```python
from build123d import *

# Parameters (mm, degrees)
F1_DEPTH = 31.75
F2_R     = 4.75
F3_DEPTH = 38.1
F5_D     = 4.572
F5_DEPTH = 7.621
F7_DEPTH = 12.7
F9_D     = 2
F11_D    = 5


# Not quite as in the source:
# - a feature names something its author has since deleted; it is built from what else it names


with BuildPart() as f1:
    # F0 (on Top) → F1 (new body)
    with BuildSketch(Plane.XY):
        with BuildLine():
            Line((-7.62, 10.9198254229), (-7.62, 0))
            ThreePointArc((-7.62, 0), (0, -7.62), (7.62, 0))
            Line((7.62, 0), (7.62, 10.9198254229))
            Line((7.62, 10.9198254229), (17.5, 10.9198254229))
            Line((17.5, 10.9198254229), (17.5, 14.0948254229))
            Line((17.5, 14.0948254229), (-17.5, 14.0948254229))
            Line((-17.5, 14.0948254229), (-17.5, 10.9198254229))
            Line((-17.5, 10.9198254229), (-7.62, 10.9198254229))
        make_face()
    extrude(amount=F1_DEPTH)

    # F2 (on face) → F3 (cut)
    with BuildSketch(Plane(origin=(0, 0, 0), x_dir=(1, 0, 0), z_dir=(0, 0, -1))):
        Circle(F2_R)
    extrude(amount=-F3_DEPTH, mode=Mode.SUBTRACT)

    # F5 (through all, one way)
    with BuildSketch(Plane(origin=(0, 0, 0), x_dir=(1, 0, 0), z_dir=(0, 1, 0))):
        with Locations((0, -14.1290773165)):
            Circle(F5_D / 2)
    extrude(amount=-F5_DEPTH, mode=Mode.SUBTRACT)

    # F6 (on face) → F7 (join)
    with BuildSketch(Plane(origin=(0, 0, 0), x_dir=(1, 0, 0), z_dir=(0, 0, -1))):
        Polygon((-7.34, -11.5548254229), (-7.34, -14.0948254229), (0, -14.0948254229), (7.34, -14.0948254229), (7.34, -11.5548254229), (0, -11.5548254229), align=None)
    extrude(amount=F7_DEPTH)

    # F9 (through all)
    with Locations(Plane.XZ.offset(-11.5548254229)):
        with Locations((0, -6.3856272027)):
            Hole(F9_D / 2)

    # F11 (through all)
    with Locations(Plane.XZ.offset(-10.9198254229)):
        with Locations((-12.9, 6.9917379814), (12.9, 6.9917379814)):
            Hole(F11_D / 2)


solid = f1.part
```
Geometry: final body of the model. Coordinates: model frame, mm. A direction names the side the tool comes from. Round coordinates to 2 decimals unless told otherwise and drop trailing zeros. Order: outer loops, then holes, each group sorted by start corner. A loop starts at its lowest first (then second) coordinate and runs counter-clockwise, first axis right, second up. Notation, with made-up numbers: (-6, 62.5) -> (27, 62.5) arc R17 cw to (27, 67.5) -> close; hole circle Ø4 at (26, 37). An arc over 180 degrees is marked (long way). Use one line per item in the form item = value.
(1) Section B-B on z = 7.5. Return loops of the section in (x, y).
Results list:
outline = (-17.5, 10.92) -> (-15.35, 10.92) -> (-15.35, 14.09) -> (-17.5, 14.09) -> close; (-10.45, 10.92) -> (-7.62, 10.92) -> (-7.62, 0) arc R7.62 ccw to (7.62, 0) -> (7.62, 10.92) -> (10.45, 10.92) -> (10.45, 14.09) -> (-10.45, 14.09) -> close; (15.35, 10.92) -> (17.5, 10.92) -> (17.5, 14.09) -> (15.35, 14.09) -> close; hole circle Ø9.5 at (0, 0)
(2) Draft query along X for faces 1 (the face through (2.18, -5.87, 13.44)), 2 (the face through (-2.763, -7.101, 15.653)), 3 (the face through (0, 6, 31.75)). Return one class per face: pulls with the +X half, pulls with the -X half, needs draft (parallel to the pull), parting line crosses it, or undercut.
Results list:
face_1 = undercut
face_2 = parting line crosses it
face_3 = needs draft
(3) First-contact query: pin 1 Ø4 at (x, y) = (-7, -0.5) entering from -Z; pin 2 Ø0.8 at (y, z) = (12.5, -7) entering from -X; pin 3 Ø4 at (y, z) = (-3, 20.5) entering from +X. Flat tips, straight axial feed; report the tip coordinate or a pass-through.
Results list:
pin_1 = 0
pin_2 = -7.34
pin_3 = 7.55
(4) Section D-D on y = 3.5. Return loops of the section in (x, z).
Results list:
outline = (-7.62, 0) -> (-3.21, 0) -> (-3.21, 31.75) -> (-7.62, 31.75) -> close; (3.21, 0) -> (7.62, 0) -> (7.62, 31.75) -> (3.21, 31.75) -> close
(5) Ray query, probe 1 along Z at (x, y) = (0, -6.9); probe 2 along Z at (x, y) = (-12.9, 12.9); probe 3 along Z at (x, y) = (-5, -3). Return the intervals inside material, ascending. Write a range as [from, to].
Results list:
probe_1 = [0, 11.84], [16.42, 31.75]
probe_2 = [0, 4.49], [9.49, 31.75]
probe_3 = [0, 31.75]
(6) Section A-A on x = -12.9. Return loops of the section in (y, z), and give its area (3 significant figures).
Results list:
outline = (10.92, 0) -> (14.09, 0) -> (14.09, 4.49) -> (10.92, 4.49) -> close; (10.92, 9.49) -> (14.09, 9.49) -> (14.09, 31.75) -> (10.92, 31.75) -> close
area = 84.9 mm^2
(7) Section C-C on x = 0. Return loops of the section in (y, z), and give its area (3 significant figures).
Results list:
outline = (-7.62, 0) -> (-4.75, 0) -> (-4.75, 11.84) -> (-7.62, 11.84) -> close; (-7.62, 16.42) -> (-4.75, 16.42) -> (-4.75, 31.75) -> (-7.62, 31.75) -> close; (4.75, 0) -> (11.55, 0) -> (11.55, -5.39) -> (14.09, -5.39) -> (14.09, 31.75) -> (4.75, 31.75) -> close; (11.55, -12.7) -> (14.09, -12.7) -> (14.09, -7.39) -> (11.55, -7.39) -> close
area = 402 mm^2
(8) Access query for faces 4 (the face through (-7.62, 6, 16)), 5 (the face through (7.34, 13, -6)), 6 (the face through (-7.34, 13, -6)). Directions: +Z, -Z, +X, -X, +Y, -Y. A direction counts if a zero-diameter tool reaches every point of the face in a straight line with its end or side. Return the directions, or none.
Results list:
face_4 = +Z, -Z, -X, -Y
face_5 = -Z, +X, +Y, -Y
face_6 = -Z, -X, +Y, -Y
